Design review of the part shown in the three views and the two pictorial views. Dimensions are in mm from the part's minimum x, y and z. Coordinates: 2 decimals unless noted, no trailing zeros. Loops run counter-clockwise (first coordinate to the right, second up) from the corner with the lowest first, then second, coordinate; pieces in that order, holes last. Notation, with made-up numbers: (31.5, -18.75) - (48.5, -18.75) arc R15 ccw to (48.5, 2.25) - close; hole circle Ø1 at (47.25, 49). An arc over 180 degrees is marked (long way). One line per question, with ' | ' between items.
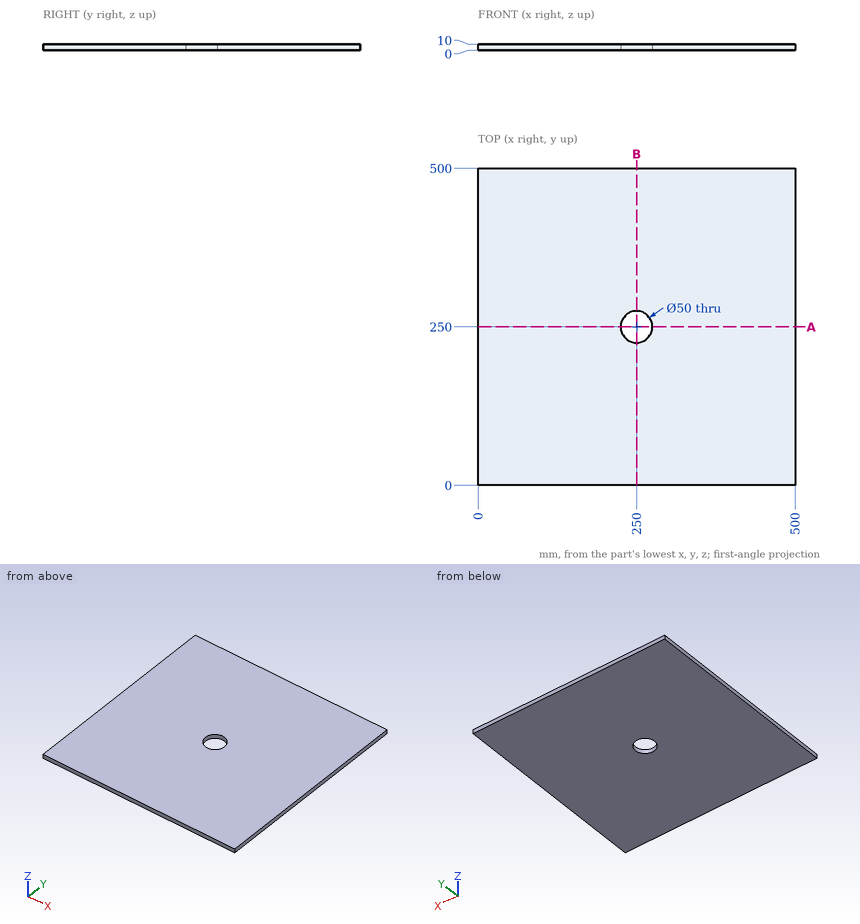
Q1. To check wall thickness, follow line 1 along Y through (x, z) = (250, 8.25); line 2 along X through (y, z) = (260.5, 3); line 3 along X through (y, z) = (267, 5.5). State the ranges of each line that lie inside material, in increasing order.
Returned:
line 1: y = 0 to 225, 275 to 500 | line 2: x = 0 to 227.31, 272.69 to 500 | line 3: x = 0 to 231.67, 268.33 to 500
Q2. Take a section at A-A (y = 250). Give the boundary of the cut face in (x, z), plus the area to 3 significant figures.
Returned:
outline: (0, 0) - (225, 0) - (225, 10) - (0, 10) - close; (275, 0) - (500, 0) - (500, 10) - (275, 10) - close | area: 4,500 mm²
